Check sheet for the modelled part. Datum: model origin and axes. Units: mm. Face numbers are marked on the shaded views. A direction names the side the tool comes from. Coordinates: 2 decimals unless noted, no trailing zeros. Loops run counter-clockwise (first coordinate to the right, second up) from the corner with the lowest first, then second, coordinate; pieces in that order, holes last. Notation, with made-up numbers: M -12,24.25 L 47,24.25 A35 cw 47,58.25 Z; hole C 11,-0.5 d7. An arc over 180 degrees is marked long. Return JSON: item names as keys, results as strings.
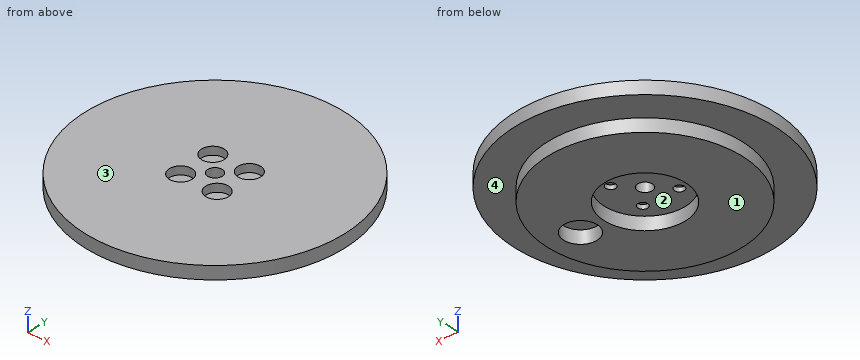
from build123d import *

# Parameters (mm, degrees)
SKETCH1_R           = 30
SKETCH1_R_2         = 12.5
BOSS_EXTRUDE1_DEPTH = 4
SKETCH2_R           = 40
SKETCH2_R_2         = 2.25
SKETCH2_R_3         = 1.5
BOSS_EXTRUDE2_DEPTH = 4
SKETCH3_R           = 3.5
CUT_EXTRUDE1_DEPTH  = 2.5
SKETCH4_R           = 5.15
CUT_EXTRUDE2_DEPTH  = 4
SKETCH5_R           = 3.5
BOSS_EXTRUDE3_DEPTH = 0.2


with BuildPart() as part:
    # Sketch1 → Boss-Extrude1 (new body)
    with BuildSketch(Plane.XY):
        Circle(SKETCH1_R)
        Circle(SKETCH1_R_2, mode=Mode.SUBTRACT)
    extrude(amount=BOSS_EXTRUDE1_DEPTH)

    # Sketch2 → Boss-Extrude2 (add)
    with BuildSketch(Plane.XY.offset(4)):
        Circle(SKETCH2_R)
        Circle(SKETCH2_R_2, mode=Mode.SUBTRACT)
        with Locations((-5.655999742, 5.657708628)):
            Circle(SKETCH2_R_3, mode=Mode.SUBTRACT)
        with Locations((-5.655999742, -5.657708628)):
            Circle(SKETCH2_R_3, mode=Mode.SUBTRACT)
        with Locations((5.655999742, -5.657708628)):
            Circle(SKETCH2_R_3, mode=Mode.SUBTRACT)
        with Locations((5.655999742, 5.657708628)):
            Circle(SKETCH2_R_3, mode=Mode.SUBTRACT)
    extrude(amount=BOSS_EXTRUDE2_DEPTH)

    # Sketch3 → Cut-Extrude1 (cut)
    with BuildSketch(Plane.XY.offset(8)):
        with Locations((-5.655999742, 5.657708628)):
            Circle(SKETCH3_R)
        with Locations((5.655999742, 5.657708628)):
            Circle(SKETCH3_R)
        with Locations((5.655999742, -5.657708628)):
            Circle(SKETCH3_R)
        with Locations((-5.655999742, -5.657708628)):
            Circle(SKETCH3_R)
    extrude(amount=-CUT_EXTRUDE1_DEPTH, mode=Mode.SUBTRACT)

    # Sketch4 → Cut-Extrude2 (cut)
    with BuildSketch(Plane(origin=(0, 0, 0), x_dir=(-1, 0, 0), z_dir=(0, 0, -1))):
        with Locations((-20, 0)):
            Circle(SKETCH4_R)
    extrude(amount=-CUT_EXTRUDE2_DEPTH, mode=Mode.SUBTRACT)

    # Sketch5 → Boss-Extrude3 (add)
    with BuildSketch(Plane.XY.offset(5.5)):
        with Locations((-5.655999742, 5.657708628)):
            Circle(SKETCH5_R)
        with Locations((5.655999742, 5.657708628)):
            Circle(SKETCH5_R)
        with Locations((-5.655999742, -5.657708628)):
            Circle(SKETCH5_R)
        with Locations((5.655999742, -5.657708628)):
            Circle(SKETCH5_R)
    extrude(amount=-BOSS_EXTRUDE3_DEPTH)


solid = part.part
1) Section check A-A on x = 0. Record the cut outline in (y, z), then the cut area to 3 significant figures.
Answers:
{"outline": "M -40,4 L -30,4 L -30,0 L -12.5,0 L -12.5,4 L -2.25,4 L -2.25,8 L -40,8 Z; M 2.25,4 L 12.5,4 L 12.5,0 L 30,0 L 30,4 L 40,4 L 40,8 L 2.25,8 Z", "area": "442 mm²"}
2) Set-up check for the marked faces 3 and 4: record each of +Z, -Z, +X, -X, +Y, -Y from which the full face is reachable in a straight line by a thin tool's end or side.
Answers:
{"face 3": "+Z, +X, -X, +Y, -Y", "face 4": "-Z"}
3) Scan lines: line 1 along Z through (x, y) = (-31.5, -8); line 2 along Y through (x, z) = (11, 1.5); line 3 along Y through (x, z) = (19.5, 1.25). Record each from-to range of solid material in increasing order. Write a range as [from, to].
Answers:
{"line 1": "[4, 8]", "line 2": "[-27.91, -5.94], [5.94, 27.91]", "line 3": "[-22.8, -5.13], [5.13, 22.8]"}
4) Section check C-C on z = 1.25. Record the cut outline in (x, y), then the cut area to 3 significant figures.
Answers:
{"outline": "C 0,0 d60; hole C 0,0 d25; hole C 20,0 d10.3", "area": "2,250 mm²"}
5) Section check B-B on y = 0. Record the cut outline in (x, z).
Answers:
{"outline": "M -40,4 L -30,4 L -30,0 L -12.5,0 L -12.5,4 L -2.25,4 L -2.25,8 L -40,8 Z; M 2.25,4 L 12.5,4 L 12.5,0 L 14.85,0 L 14.85,4 L 25.15,4 L 25.15,0 L 30,0 L 30,4 L 40,4 L 40,8 L 2.25,8 Z"}
6) Section check D-D on x = 22.5. Record the cut outline in (y, z).
Answers:
{"outline": "M -33.07,4 L -19.84,4 L -19.84,0 L -4.5,0 L -4.5,4 L 4.5,4 L 4.5,0 L 19.84,0 L 19.84,4 L 33.07,4 L 33.07,8 L -33.07,8 Z"}
7) Draft check along X on the marked faces 1 and 2. Enter one of: +X half, -X half, draft (parallel to the pull), parting line (faces both ways), or undercut.
Answers:
{"face 1": "draft", "face 2": "undercut"}
8) Go/stop test with flat-tipped pins: pin 1 Ø2 at (x, y) = (-4.5, 4) entering from +Z; pin 2 Ø0.9 at (x, y) = (-5.5, 5.5) entering from -Z; pin 3 Ø2.5 at (x, y) = (5.5, -6) entering from -Z; pin 4 Ø3.5 at (x, y) = (0, 0) entering from -Z. Record where each tip stops, or that it passes through.
Answers:
{"pin 1": "z = 5.5", "pin 2": "z = 5.3", "pin 3": "z = 4", "pin 4": "through"}
